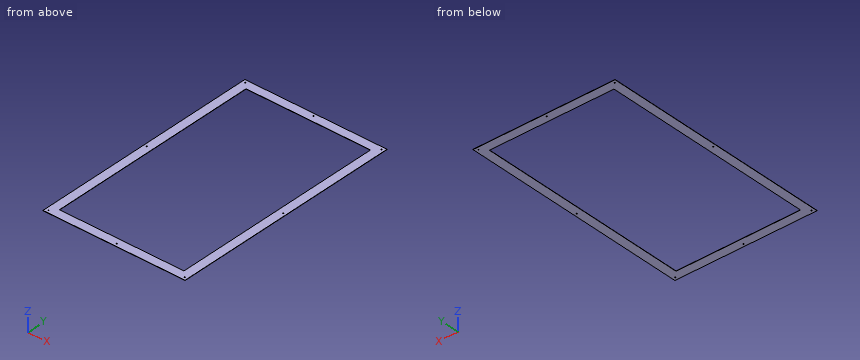
```python
from build123d import *

# Parameters (mm, degrees)
F0_W     = 617.5375
F0_H     = 1008.0625
F0_W_2   = 541.3375
F0_H_2   = 931.8625
F1_DEPTH = 1.21412
F3_D     = 4.7625


with BuildPart() as f1:
    # F0 (on Top) → F1 (new body)
    with BuildSketch(Plane.XY):
        Rectangle(F0_W, F0_H)
        Rectangle(F0_W_2, F0_H_2, mode=Mode.SUBTRACT)
    extrude(amount=F1_DEPTH)

    # F3 (through all)
    with Locations(Plane(origin=(0, 0, 0), x_dir=(1, 0, 0), z_dir=(0, 0, -1))):
        with Locations((-296.06875, 491.33125), (0, 491.33125), (296.06875, 491.33125), (296.06875, 0), (296.06875, -491.33125), (0, -491.33125), (-296.06875, -491.33125), (-296.06875, 0)):
            Hole(F3_D / 2)


solid = f1.part
```
For this review, take the finished solid that the model builds, in its own axes (mm). Round coordinates to 2 decimals unless told otherwise and drop trailing zeros. Loops run counter-clockwise (first coordinate to the right, second up) from the corner with the lowest first, then second, coordinate; pieces in that order, holes last.
(1) Wall thickness on line 1 along Y through (x, z) = (0, 0.45); line 2 along Y through (x, z) = (44, 1.15); line 3 along X through (y, z) = (246.5, 0.95): over which ranges is each line inside the solid? List them lowest first.
Returned:
line 1: y = -504.03 to -493.71, -488.95 to -465.93, 465.93 to 488.95, 493.71 to 504.03
line 2: y = -504.03 to -465.93, 465.93 to 504.03
line 3: x = -308.77 to -270.67, 270.67 to 308.77
(2) We need section A-A (x = -128). Give the boundary of the cut face in (y, z), plus the area to 3 significant figures.
Returned:
outline: (-504.03, 0) - (-465.93, 0) - (-465.93, 1.21) - (-504.03, 1.21) - close; (465.93, 0) - (504.03, 0) - (504.03, 1.21) - (465.93, 1.21) - close
area: 92.5 mm2
(3) We need section B-B (y = -281.5). Give the boundary of the cut face in (x, z).
Returned:
outline: (-308.77, 0) - (-270.67, 0) - (-270.67, 1.21) - (-308.77, 1.21) - close; (270.67, 0) - (308.77, 0) - (308.77, 1.21) - (270.67, 1.21) - close
(4) We need section C-C (z = 0.95). State how many separate pieces and enclosed holes the cut face has, plus the area to 3 significant figures.
Returned:
separate pieces: 1
enclosed holes: 9
area: 118,000 mm2
(5) Clearance check with a flat-ended pin moving along its axis: P1, Ø4, axis at x = 296.07, y = -491.33, coming from the +Z side. State where the tip first meets the part, or that it passes through.
Returned:
P1: passes through
